Autodesk Inventor part; units mm, degrees
ref_plane "YZ Plane" through (0, 0, 0) normal (1, 0, 0) x (0, 1, 0)
ref_plane "XZ Plane" through (0, 0, 0) normal (0, 1, 0) x (-1, 0, 0)
ref_plane "XY Plane" through (0, 0, 0) normal (0, 0, 1) x (1, 0, 0)
sketch "Sketch1" plane through (0, 0, 0) normal (0, 0, 1) x (1, 0, 0)
  line L0 (0, 0) -> (342.9, 0)
  line L1 (342.9, 0) -> (342.9, -180.975)
  line L2 (342.9, -180.975) -> (0, -180.975)
  line L3 (0, -180.975) -> (0, 0)
  line L4 (342.9, -88.9) -> (381, -88.9)
  line L5 (381, -88.9) -> (381, -146.05)
  line L6 (381, -146.05) -> (342.9, -146.05)
  line L7 (342.9, -146.05) -> (342.9, -88.9)
  line L8 (381, -146.05) -> (342.9, -180.975)
  line L9 (381, -88.9) -> (342.9, 0)
  dimension "d0" = 342.9
  dimension "d1" = 180.975
  dimension "d2" = 88.9
  dimension "d3" = 34.925
  dimension "d4" = 38.1
extrude "Extrusion1" add sketch "Sketch1" along normal blind 209.55
shell "Shell1" thickness 19.05 removed faces 2 at (228.6, 0, 69.85) at (355.6, -29.6333, 139.7) ; own thickness 19.05 on faces at (114.3, -60.325, 209.55) (381, -127, 69.85) (114.3, -60.325, 0) ; own thickness 12.7 on faces at (0, -60.325, 69.85) ; own thickness 3.175 on faces at (114.3, -180.975, 69.85) (355.6, -169.3333, 69.85)
hole "Hole1" at (0, -63.5, 166.6875) direction (1, 0, 0) diameter 11.1125 end up to surface
properties part number "bin" material "Thermoplastic Resin"
The model under review builds one solid part; all positions refer to its coordinate system, in mm. A direction names the side the tool comes from. Round coordinates to 2 decimals unless told otherwise and drop trailing zeros. Loops run counter-clockwise (first coordinate to the right, second up) from the corner with the lowest first, then second, coordinate; pieces in that order, holes last. Notation, with made-up numbers: M 62,56.5 L 107,56.5 A27 cw 107,74.5 Z; hole C 86.5,-17.5 d3. An arc over 180 degrees is marked long. Put each result on its own line as item: value.
Q1. Consider section A-A, the plane z = 116. Give the boundary of the cut face in (x, y) (3 decimals), then the cut area to 3 significant figures.
Result set:
outline: M 0,-180.975 L 342.9,-180.975 L 381,-146.05 L 381,-88.9 L 361.95,-44.45 L 361.95,-159.205 L 341.665,-177.8 L 12.7,-177.8 L 12.7,0 L 0,0 Z
area: 5,110 mm²
Q2. To check wall thickness, follow L1, parallel to Z at x = 324, y = -170; L2, parallel to Z at x = 5.5, y = -63.5; L3, parallel to X at y = -112, z = 26. State the ranges of each line that lie inside material, in increasing order.
Result set:
L1: z = 0 to 19.05, 190.5 to 209.55
L2: z = 0 to 161.13, 172.24 to 209.55
L3: x = 0 to 12.7, 361.95 to 381
Q3. Consider section B-B, the plane x = 82.5. Give the boundary of the cut face in (y, z) (3 decimals).
Result set:
outline: M -180.975,0 L 0,0 L 0,19.05 L -177.8,19.05 L -177.8,190.5 L 0,190.5 L 0,209.55 L -180.975,209.55 Z
Q4. Mouldability with a two-part tool opening along Z and no side actions: class faces 3 (the flat face through (188, -89, 209.55)), 4 (the flat face through (174, -180.975, 103)), 5 (the flat face through (185, -88, 19.05)), 6 (the cylindrical face through (6.439, -58.076, 165.483)) as released by +Z, released by -Z, zero draft, split by the parting line, or undercut.
Result set:
face 3: released by +Z
face 4: zero draft
face 5: undercut
face 6: undercut
Q5. Machinability: for faces 1 (the flat face through (361.95, -101, 104)), 2 (the flat face through (0, -92, 103)), which of the approach directions +Z, -Z, +X, -X, +Y, -Y give a long, thin tool a straight path to every point of the face, cutting with its end or side? Answer none if there is none.
Result set:
face 1: +Y
face 2: +Z, -Z, -X, +Y, -Y
Q6. For pin 1 (6 mm diameter, centred on x = 118, z = 140.5, fed in from +Y); pin 2 (6 mm diameter, centred on y = -102.5, z = 149, fed in from -X); pin 3 (10 mm diameter, centred on y = -56.5, z = 130, fed in from +X); pin 4 (5 mm diameter, centred on y = -158, z = 103, fed in from +X), all flat-tipped, find the tip position at first contact; note any pin that passes through.
Result set:
pin 1: stops at y = -177.8
pin 2: stops at x = 0
pin 3: stops at x = 369.26
pin 4: stops at x = 370.69
Q7. Consider section C-C, the plane y = -77.5. Give the boundary of the cut face in (x, z).
Result set:
outline: M 0,0 L 376.11,0 L 376.11,209.55 L 0,209.55 Z; hole M 12.7,19.05 L 361.95,19.05 L 361.95,190.5 L 12.7,190.5 Z
Q8. Consider section D-D, the plane y = -16. Give the boundary of the cut face in (x, z).
Result set:
outline: M 0,0 L 349.76,0 L 349.76,19.05 L 12.7,19.05 L 12.7,190.5 L 349.76,190.5 L 349.76,209.55 L 0,209.55 Z
